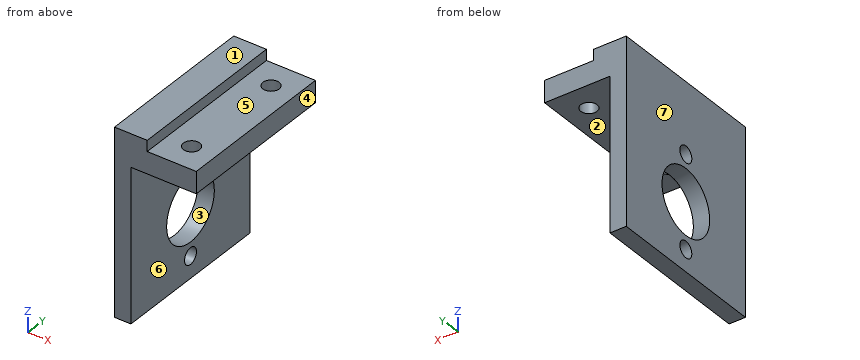
from build123d import *

# Parameters (mm, degrees)
EXTRUDE_1_DEPTH     = 30
SKETCH_2_R          = 6
CUT_EXTRUDE_1_DEPTH = 26
SKETCH_3_W          = 6
SKETCH_3_H          = 30
EXTRUDE_2_DEPTH     = 2
SKETCH_4_R          = 1.5
CUT_EXTRUDE_2_DEPTH = 46.475268004
SKETCH_5_R          = 1.5
CUT_EXTRUDE_3_DEPTH = 47.357307946


with BuildPart() as part:
    # 草图1 → 凸台-拉伸1 (new body)
    with BuildSketch(Plane(origin=(0, 0, 0), x_dir=(1, 0, 0), z_dir=(0, 1, 0))):
        Polygon((0, 0), (15, 0), (15, 4), (3, 4), (3, 32), (0, 32), align=None)
    extrude(amount=EXTRUDE_1_DEPTH)

    # 草图2 → 切除-拉伸1 (cut)
    with BuildSketch(Plane(origin=(3, 0, 0), x_dir=(0, 0, -1), z_dir=(1, 0, 0))):
        with Locations((19.5, 15)):
            Circle(SKETCH_2_R)
    extrude(amount=-CUT_EXTRUDE_1_DEPTH, mode=Mode.SUBTRACT)

    # 草图3 → 凸台-拉伸2 (add)
    with BuildSketch(Plane.XY):
        with Locations((3, 15)):
            Rectangle(SKETCH_3_W, SKETCH_3_H)
    extrude(amount=EXTRUDE_2_DEPTH)

    # 草图4 → 切除-拉伸2 (cut, through all)
    with BuildSketch(Plane(origin=(3, 0, 0), x_dir=(0, 0, -1), z_dir=(1, 0, 0))):
        with Locations((28, 15)):
            Circle(SKETCH_4_R)
        with Locations((11, 15)):
            Circle(SKETCH_4_R)
    extrude(amount=-CUT_EXTRUDE_2_DEPTH, mode=Mode.SUBTRACT)

    # 草图5 → 切除-拉伸3 (cut, through all)
    with BuildSketch(Plane.XY):
        with Locations((10.5, 25)):
            Circle(SKETCH_5_R)
        with Locations((10.5, 5)):
            Circle(SKETCH_5_R)
    extrude(amount=-CUT_EXTRUDE_3_DEPTH, mode=Mode.SUBTRACT)


solid = part.part
Model file for the job. Use its own axes, mm. Face numbers are marked on the shaded views. A direction names the side the tool comes from. Give positions to 0.01 mm unless a question says otherwise; leave off trailing zeros. Loops run counter-clockwise (first coordinate to the right, second up) from the corner with the lowest first, then second, coordinate; pieces in that order, holes last.
1) Saw through at C-C (y = 5). Write the cut outline in (x, z).
2) Saw through at D-D (x = 1.75). Write the cut outline in (y, z).
3) Saw through at B-B (z = -28). Write the cut outline in (x, y), plus the area to 3 significant figures.
4) Saw through at A-A (y = 15). Write the cut outline in (x, z), plus the area to 3 significant figures.
5) Flat gauge pins, fed straight in: pin 1 Ø7 at (y, z) = (15, -19.5) entering from +X; pin 2 Ø2 at (y, z) = (26, -7) entering from +X; pin 3 Ø4 at (y, z) = (15, -28) entering from -X; pin 4 Ø1 at (x, y) = (6.5, 14.5) entering from -Z. Where does each tip first touch, or does it go through?
6) Tool access for the marked faces 5, 6 and 7: list every direction of +Z, -Z, +X, -X, +Y, -Y with a clear straight run to the whole face (end or side of a thin tool).
7) Pull direction Z, two halves, no side cores. Call the marked faces 1, 2, 3 and 4: +Z half, -Z half, draft (parallel to the pull), parting line (faces both ways), or undercut.
8) Wall check: line 1 (Y direction, x = 10.5, z = -2.5); line 2 (Y direction, x = 9.75, z = -0.5); line 3 (Y direction, x = 0.75, z = -19.5). Give the ranges that are in metal, low to high.
Answer block:
1. outline: (0, -32) - (3, -32) - (3, -4) - (9, -4) - (9, 0) - (6, 0) - (6, 2) - (0, 2) - close; (12, -4) - (15, -4) - (15, 0) - (12, 0) - close
2. outline: (0, -32) - (30, -32) - (30, 2) - (0, 2) - close; hole circle Ø12 at (15, -19.5); hole circle Ø3 at (15, -28); hole circle Ø3 at (15, -11)
3. outline: (0, 0) - (3, 0) - (3, 13.5) - (0, 13.5) - close; (0, 16.5) - (3, 16.5) - (3, 30) - (0, 30) - close
3. area: 81.0 mm2
4. outline: (0, -32) - (3, -32) - (3, -29.5) - (0, -29.5) - close; (0, -26.5) - (3, -26.5) - (3, -25.5) - (0, -25.5) - close; (0, -13.5) - (3, -13.5) - (3, -12.5) - (0, -12.5) - close; (0, -9.5) - (3, -9.5) - (3, -4) - (15, -4) - (15, 0) - (6, 0) - (6, 2) - (0, 2) - close
4. area: 102 mm2
5. pin 1: passes through
5. pin 2: stops at x = 3
5. pin 3: stops at x = 0
5. pin 4: stops at z = -4
6. face 5: +Z, +X, +Y, -Y
6. face 6: -Z, +X, +Y, -Y
6. face 7: +Z, -Z, -X, +Y, -Y
7. face 1: +Z half
7. face 2: -Z half
7. face 3: undercut
7. face 4: draft
8. line 1: y = 0 to 3.5, 6.5 to 23.5, 26.5 to 30
8. line 2: y = 0 to 3.7, 6.3 to 23.7, 26.3 to 30
8. line 3: y = 0 to 9, 21 to 30
